Input: part model. Units: mm. Frame: model coordinates. A direction names the side the tool comes from. Give positions to 0.01 mm unless a question says otherwise; leave off trailing zeros. Loops run counter-clockwise (first coordinate to the right, second up) from the corner with the lowest first, then second, coordinate; pieces in that order, holes last. Notation, with made-up numbers: (38.5, 23) -> (45.5, 23) arc R18 cw to (45.5, 54) -> close; hole circle Ø7 at (-10.5, 57.5). An arc over 180 degrees is marked (long way). Answer as a JSON object with one key per item and string values.
Autodesk Inventor part; units mm, degrees
ref_plane "YZ Plane" through (0, 0, 0) normal (1, 0, 0) x (0, 1, 0)
ref_plane "XZ Plane" through (0, 0, 0) normal (0, 1, 0) x (-1, 0, 0)
ref_plane "XY Plane" through (0, 0, 0) normal (0, 0, 1) x (1, 0, 0)
sketch "Эскиз1" plane through (0, 0, 0) normal (0, 1, 0) x (-1, 0, 0)
  line L0 (-15, 20) -> (15, 20)
  line L1 (15, 20) -> (15, -20)
  line L2 (15, -20) -> (-15, -20)
  line L3 (-15, -20) -> (-15, 20)
  line L4 (-15, 20) -> (15, -20) construction
  line L5 (15, 20) -> (-15, -20) construction
  point P0 (0, 0)
  dimension "d0" = 40
  dimension "d1" = 30
extrude "Выдавливание1" add sketch "Эскиз1" along normal blind 6
sketch "Эскиз2" plane through (-15, 0, 20) normal (0, 0, 1) x (1, 0, 0)
  line L0 (30, 0) -> (0, 0)
  line L1 (0, 0) -> (30, 0)
  line L2 (30, 0) -> (30, 19)
  line L3 (30, 19) -> (0, 19)
  line L4 (0, 19) -> (0, 0)
  line L5 (0, 6) -> (30, 6)
  point P0 (15, 0)
  dimension "d4" = 13
extrude "Выдавливание2" add sketch "Эскиз2" along normal blind 3
sketch "Эскиз4" plane through (-15, 19, 20) normal (0, 1, 0) x (1, 0, 0)
  line L0 (0, 40) -> (0, 0)
  line L1 (0, 0) -> (30, 0)
  line L2 (30, 0) -> (30, -15)
  line L3 (30, -15) -> (0, -15)
  line L4 (0, -15) -> (0, 0)
  point P0 (15, 20)
  point P1 (30, 0)
  dimension "d7" = 15
extrude "Выдавливание3" add sketch "Эскиз4" against normal blind 3
fillet "Сопряжение1" radius 3 3 edges at (15, 17.5, 35) (-15, 17.5, 35) (0, 0, 23)
sketch "Эскиз5" plane through (-15, 19, 20) normal (0, 1, 0) x (1, 0, 0)
  circle A0 centre (8, -9) radius 1.65
  circle A1 centre (22, -9) radius 1.65
  line L0 (0, 0) -> (0, -12)
  line L1 (30, -3) -> (30, -12)
  line L2 (30, 0) -> (0, 0)
  point P0 (15, 20)
  dimension "d11" = 3.3
  dimension "d12" = 3.3
  dimension "d13" = 8
  dimension "d14" = 8
  dimension "d15" = 9
  dimension "d16" = 9
extrude "Выдавливание4" cut sketch "Эскиз5" against normal blind 3
sketch "Эскиз6" plane through (-15, 16, 20) normal (0, -1, 0) x (1, 0, 0)
  circle A0 centre (22, 9) radius 1.65 construction
  circle A1 centre (8, 9) radius 1.65 construction
  line L0 (24.75, 7.4123) -> (22, 5.8246)
  line L1 (22, 5.8246) -> (19.25, 7.4123)
  line L2 (19.25, 7.4123) -> (19.25, 10.5877)
  line L3 (19.25, 10.5877) -> (22, 12.1754)
  line L4 (22, 12.1754) -> (24.75, 10.5877)
  line L5 (24.75, 10.5877) -> (24.75, 7.4123)
  line L6 (10.75, 7.4123) -> (8, 5.8246)
  line L7 (8, 5.8246) -> (5.25, 7.4123)
  line L8 (5.25, 7.4123) -> (5.25, 10.5877)
  line L9 (5.25, 10.5877) -> (8, 12.1754)
  line L10 (8, 12.1754) -> (10.75, 10.5877)
  line L11 (10.75, 10.5877) -> (10.75, 7.4123)
  line L12 (0, 12) -> (0, 3)
  line L13 (30, 3) -> (30, 12)
  point P0 (15, -20)
  point P1 (19.25, 9)
  dimension "d19" = 5.5
  dimension "d20" = 5.5
extrude "Выдавливание5" cut sketch "Эскиз6" against normal blind 2.2
mirror "Зеркальное отражение1" about plane through (0, 0, 0) normal (0, 0, 1) of "Выдавливание2", "Сопряжение1", "Выдавливание5", "Выдавливание4", "Выдавливание3"
sketch "Эскиз7" plane through (0, 0, 0) normal (0, -1, 0) x (1, 0, 0)
  circle A0 centre (0, 12) radius 2.1
  circle A1 centre (0, -12) radius 2.1
  point P0 (0, 0)
  dimension "d23" = 4.2
  dimension "d24" = 4.2
  dimension "d25" = 12
  dimension "d26" = 12
extrude "Выдавливание6" cut sketch "Эскиз7" against normal blind 5
sketch "Эскиз8" plane through (0, 5, 12) normal (0, -1, 0) x (1, 0, 0)
  circle A0 centre (0, 0) radius 1.6
  circle A1 centre (0, -24) radius 2.1
  circle A2 centre (0, -24) radius 1.6
  point P0 (0, -12)
  dimension "d29" = 3.2
  dimension "d30" = 3.2
extrude "Выдавливание7" cut sketch "Эскиз8" against normal blind 6 contours A0 | A2
properties part number "креп_камеры_ros"
Q1. Access query for faces 4 (the flat face through (0, 10, 23)), 5 (the flat face through (-5.64, 17.08, -26.61)), 6 (the flat face through (0, 10, -23)). Directions: +Z, -Z, +X, -X, +Y, -Y. A direction counts if a zero-diameter tool reaches every point of the face in a straight line with its end or side. Return the directions, or none.
Evaluation:
{"face 4": "+Z, +X, -X, -Y", "face 5": "-Y", "face 6": "-Z, +X, -X, -Y"}
Q2. Section A-A, the plane z = -29. Return the cut outline in (x, y), then the cut area to 3 significant figures.
Evaluation:
{"outline": "(-15, 16) -> (-9.75, 16) -> (-9.75, 18.2) -> (-8.65, 18.2) -> (-8.65, 19) -> (-15, 19) -> close; (-5.35, 18.2) -> (-4.25, 18.2) -> (-4.25, 16) -> (4.25, 16) -> (4.25, 18.2) -> (5.35, 18.2) -> (5.35, 19) -> (-5.35, 19) -> close; (8.65, 18.2) -> (9.75, 18.2) -> (9.75, 16) -> (15, 16) -> (15, 19) -> (8.65, 19) -> close", "area": "60.5 mm2"}
Q3. Draft query along Z for faces 1 (the flat face through (-8.394, 17.085, 31.37)), 2 (the flat face through (0, 16, 29)), 3 (the cylindrical face through (14.14, 17.48, 34.1)). Return one class per face: +Z half, -Z half, draft (parallel to the pull), parting line (faces both ways), or undercut.
Evaluation:
{"face 1": "undercut", "face 2": "draft", "face 3": "+Z half"}
Q4. Ray query, line 1 along Z through (x, y) = (0, 5.65); line 2 along X through (y, z) = (18.65, -29); line 3 along Z through (x, y) = (7, 18.4). Return the intervals inside material, ascending.
Evaluation:
{"line 1": "z = -23 to -13.6, -10.4 to 10.4, 13.6 to 23", "line 2": "x = -15 to -8.65, -5.35 to 5.35, 8.65 to 15", "line 3": "z = -35 to -30.65, -27.35 to -20, 20 to 27.35, 30.65 to 35"}
Q5. Section D-D, the plane z = -12. Return the cut outline in (x, y), then the cut area to 3 significant figures.
Evaluation:
{"outline": "(-15, 0) -> (-2.1, 0) -> (-2.1, 5) -> (-1.6, 5) -> (-1.6, 6) -> (-15, 6) -> close; (1.6, 5) -> (2.1, 5) -> (2.1, 0) -> (15, 0) -> (15, 6) -> (1.6, 6) -> close", "area": "156 mm2"}
Q6. Section C-C, the plane x = 0. Give the number of separate pieces and of enclosed holes in the cut face, then the cut area to 3 significant figures.
Evaluation:
{"separate pieces": "3", "enclosed holes": "0", "area": "374 mm2"}
Q7. Section B-B, the plane y = 10.5. Return the cut outline in (x, z).
Evaluation:
{"outline": "(-15, -23) -> (15, -23) -> (15, -20) -> (-15, -20) -> close; (-15, 20) -> (15, 20) -> (15, 23) -> (-15, 23) -> close"}
Q8. Pin query (flat end, axial travel): pin 1 (5 mm diameter, centred on x = 0, z = 12, fed in from -Y); pin 2 (6.5 mm diameter, centred on x = -3, y = 10.5, fed in from -Z); pin 3 (3.5 mm diameter, centred on x = 7.5, z = -26.5, fed in from -Y); pin 4 (3 mm diameter, centred on x = 1.5, y = 10, fed in from +Z). Return the tip coordinate at first contact, or that it passes through.
Evaluation:
{"pin 1": "stops at y = 0", "pin 2": "stops at z = -23", "pin 3": "stops at y = 16", "pin 4": "stops at z = 23"}
